Part model, mm, in its own coordinate system. A direction names the side the tool comes from. Give positions to 0.01 mm unless a question says otherwise; leave off trailing zeros. Order: outer loops, then holes, each group sorted by start corner. A loop starts at its lowest first (then second) coordinate and runs counter-clockwise, first axis right, second up. Notation, with made-up numbers: (7, 7) - (28, 7) arc R21 ccw to (28, 24) - close; hole circle Ø8 at (-27.75, 85). An arc over 180 degrees is marked (long way). One line per item, written item: value.
```python
from build123d import *

# Parameters (mm, degrees)
SKETCH1_R                = 24.5
SKETCH1_R_2              = 22
BOSS_EXTRUDE1_DEPTH      = 1
BOSS_EXTRUDE2_DEPTH      = 1
SKETCH3_R                = 7
CUT_EXTRUDE1_DEPTH       = 0.9
FILLET1_R                = 0.5
BOSS_EXTRUDE3_DEPTH      = 4
BOSS_EXTRUDE3_DEPTH_BACK = 21.5
SKETCH4_R                = 28.5
SKETCH4_R_2              = 24.5
BOSS_EXTRUDE4_DEPTH      = 8
SKETCH6_R                = 4.6
BOSS_EXTRUDE5_DEPTH      = 17.5


with BuildPart() as part:
    # Sketch1 → Boss-Extrude1 (new body)
    with BuildSketch(Plane.XY):
        Circle(SKETCH1_R)
        Circle(SKETCH1_R_2, mode=Mode.SUBTRACT)
    extrude(amount=BOSS_EXTRUDE1_DEPTH)

    # Sketch2 → Boss-Extrude2 (add)
    with BuildSketch(Plane.XY.offset(1)):
        with BuildLine():
            Line((-1.614189839, 23), (1.614189839, 23))
            ThreePointArc((1.614189839, 23), (2.986252504, 22.455143994), (3.610738586, 21.117444044))
            Line((3.610738586, 21.117444044), (4.203159318, 11.046291601))
            ThreePointArc((4.203159318, 11.046291601), (5.845115801, 8.045111712), (9.206799949, 7.410933888))
            Line((9.206799949, 7.410933888), (18.96810318, 9.959665548))
            ThreePointArc((18.96810318, 9.959665548), (20.433308247, 9.779116009), (21.375487782, 8.642576636))
            Line((21.375487782, 8.642576636), (22.373111967, 5.572205105))
            ThreePointArc((22.373111967, 5.572205105), (22.278913793, 4.098926202), (21.199662351, 3.091632627))
            Line((21.199662351, 3.091632627), (11.804495268, -0.583950228))
            ThreePointArc((11.804495268, -0.583950228), (9.457596034, -3.072959231), (9.893274614, -6.46608257))
            Line((9.893274614, -6.46608257), (15.333671053, -14.962032219))
            ThreePointArc((15.333671053, -14.962032219), (15.614731503, -16.411317921), (14.824967815, -17.658593889))
            Line((14.824967815, -17.658593889), (12.213153791, -19.556187853))
            ThreePointArc((12.213153791, -19.556187853), (10.782873453, -19.921868284), (9.491373297, -19.20671))
            Line((9.491373297, -19.20671), (3.092419978, -11.40719269))
            ThreePointArc((3.092419978, -11.40719269), (0, -9.944304962), (-3.092419978, -11.40719269))
            Line((-3.092419978, -11.40719269), (-9.491373297, -19.20671))
            ThreePointArc((-9.491373297, -19.20671), (-10.782873453, -19.921868284), (-12.213153791, -19.556187853))
            Line((-12.213153791, -19.556187853), (-14.824967815, -17.658593889))
            ThreePointArc((-14.824967815, -17.658593889), (-15.614731503, -16.411317921), (-15.333671053, -14.962032219))
            Line((-15.333671053, -14.962032219), (-9.893274614, -6.46608257))
            ThreePointArc((-9.893274614, -6.46608257), (-9.457596034, -3.072959231), (-11.804495268, -0.583950228))
            Line((-11.804495268, -0.583950228), (-21.199662351, 3.091632627))
            ThreePointArc((-21.199662351, 3.091632627), (-22.278913793, 4.098926202), (-22.373111967, 5.572205105))
            Line((-22.373111967, 5.572205105), (-21.375487782, 8.642576636))
            ThreePointArc((-21.375487782, 8.642576636), (-20.433308247, 9.779116009), (-18.96810318, 9.959665548))
            Line((-18.96810318, 9.959665548), (-9.206799949, 7.410933888))
            ThreePointArc((-9.206799949, 7.410933888), (-5.845115801, 8.045111712), (-4.203159318, 11.046291601))
            Line((-4.203159318, 11.046291601), (-3.610738586, 21.117444044))
            ThreePointArc((-3.610738586, 21.117444044), (-2.986252504, 22.455143994), (-1.614189839, 23))
        make_face()
    extrude(amount=BOSS_EXTRUDE2_DEPTH)

    # Sketch3 → Cut-Extrude1 (cut)
    with BuildSketch(Plane.XY.offset(2)):
        Circle(SKETCH3_R)
    extrude(amount=-CUT_EXTRUDE1_DEPTH, mode=Mode.SUBTRACT)

    # Fillet1
    fillet1_edges = [part.edges().sort_by_distance(p)[0] for p in [
        (-7, 0, 1.1),
    ]]
    fillet(fillet1_edges, radius=FILLET1_R)

    # Sketch4 → Boss-Extrude3 (add, two sides: drawn at the far end of the back side and taken through both)
    with BuildSketch(Plane.XY.offset(-BOSS_EXTRUDE3_DEPTH_BACK)):
        Circle(SKETCH4_R)
        Circle(SKETCH4_R_2, mode=Mode.SUBTRACT)
    extrude(amount=BOSS_EXTRUDE3_DEPTH + BOSS_EXTRUDE3_DEPTH_BACK)

    # Sketch5 → Boss-Extrude4 (add)
    with BuildSketch(Plane(origin=(0, 0, 1), x_dir=(-1, 0, 0), z_dir=(0, 0, -1))):
        with BuildLine():
            Line((22.451817346, 7.975399256), (22.851723851, 6.744613588))
            Line((22.851723851, 6.744613588), (7.30628104, 1.693593032))
            ThreePointArc((7.30628104, 1.693593032), (7.132923872, -2.317627458), (4.915436519, -5.664669789))
            Line((4.915436519, -5.664669789), (14.523048547, -18.888413283))
            Line((14.523048547, -18.888413283), (13.476079724, -19.649080658))
            Line((13.476079724, -19.649080658), (3.868467697, -6.425337165))
            ThreePointArc((3.868467697, -6.425337165), (0, -7.5), (-3.868467697, -6.425337165))
            Line((-3.868467697, -6.425337165), (-13.476079724, -19.649080658))
            Line((-13.476079724, -19.649080658), (-14.523048547, -18.888413283))
            Line((-14.523048547, -18.888413283), (-4.915436519, -5.664669789))
            ThreePointArc((-4.915436519, -5.664669789), (-7.132923872, -2.317627458), (-7.30628104, 1.693593032))
            Line((-7.30628104, 1.693593032), (-22.851723851, 6.744613588))
            Line((-22.851723851, 6.744613588), (-22.451817346, 7.975399256))
            Line((-22.451817346, 7.975399256), (-6.906374535, 2.9243787))
            ThreePointArc((-6.906374535, 2.9243787), (-4.408389392, 6.067627458), (-0.647062318, 7.472035222))
            Line((-0.647062318, 7.472035222), (-0.647062318, 23.817481096))
            Line((-0.647062318, 23.817481096), (0.647062318, 23.817481096))
            Line((0.647062318, 23.817481096), (0.647062318, 7.472035222))
            ThreePointArc((0.647062318, 7.472035222), (4.408389392, 6.067627458), (6.906374535, 2.9243787))
            Line((6.906374535, 2.9243787), (22.451817346, 7.975399256))
        make_face()
    extrude(amount=BOSS_EXTRUDE4_DEPTH)

    # Sketch6 → Boss-Extrude5 (add)
    with BuildSketch(Plane(origin=(0, 0, -7), x_dir=(-1, 0, 0), z_dir=(0, 0, -1))):
        Circle(SKETCH6_R)
        with BuildLine():
            Line((-2.436698586, -1.75), (2.436698586, -1.75))
            ThreePointArc((2.436698586, -1.75), (3, 0), (2.436698586, 1.75))
            Line((2.436698586, 1.75), (-2.436698586, 1.75))
            ThreePointArc((-2.436698586, 1.75), (-3, 0), (-2.436698586, -1.75))
        make_face(mode=Mode.SUBTRACT)
    extrude(amount=BOSS_EXTRUDE5_DEPTH)


solid = part.part
```
1) Wall check: line 1 along Y through (x, z) = (0, 1.7); line 2 along Y through (x, z) = (0, -10); line 3 along Y through (x, z) = (0, -6). Give the ranges that are in metal, low to high. Write a range as [from, to].
Answer:
line 1: y = [-28.5, -24.5], [-9.94, -7], [7, 23], [24.5, 28.5]
line 2: y = [-28.5, -24.5], [-4.6, -1.75], [1.75, 4.6], [24.5, 28.5]
line 3: y = [-28.5, -24.5], [-7.5, 23.82], [24.5, 28.5]
2) Two-plate mould, pull along Y, no slides. Class faces 1 (the face through (13, 21, -21.5)), 2 (the face through (0, 0, -7)): pulls with the +Y half, pulls with the -Y half, needs draft (parallel to the pull), parting line crosses it, or undercut.
Answer:
face 1: needs draft
face 2: undercut
3) Slice it at D-D on y = 17. Write the cut outline in (x, z).
Answer:
outline: (-22.87, -21.5) - (-17.64, -21.5) - (-17.64, 0) - (-13.96, 0) - (-13.96, 1) - (-17.64, 1) - (-17.64, 4) - (-22.87, 4) - close; (-3.85, 1) - (-0.65, 1) - (-0.65, -7) - (0.65, -7) - (0.65, 1) - (3.85, 1) - (3.85, 2) - (-3.85, 2) - close; (13.96, 0) - (17.64, 0) - (17.64, -21.5) - (22.87, -21.5) - (22.87, 4) - (17.64, 4) - (17.64, 1) - (13.96, 1) - close
4) Slice it at A-A on z = -2.5. Write the cut outline in (x, y).
Answer:
outline: circle Ø57 at (0, 0); (-22.85, 6.74) - (-7.31, 1.69) arc R7.5 ccw to (-4.92, -5.66) - (-14.52, -18.89) - (-13.48, -19.65) - (-3.87, -6.43) arc R7.5 ccw to (3.87, -6.43) - (13.48, -19.65) - (14.52, -18.89) - (4.92, -5.66) arc R7.5 ccw to (7.31, 1.69) - (22.85, 6.74) - (22.45, 7.98) - (6.91, 2.92) arc R7.5 ccw to (0.65, 7.47) - (0.65, 23.82) - (-0.65, 23.82) - (-0.65, 7.47) arc R7.5 ccw to (-6.91, 2.92) - (-22.45, 7.98) - close; hole circle Ø49 at (0, 0)
5) Slice it at B-B on z = -18.5. Write the cut outline in (x, y), then the cut area to 3 significant figures.
Answer:
outline: circle Ø57 at (0, 0); circle Ø9.2 at (0, 0); hole circle Ø49 at (0, 0); hole (-2.44, -1.75) - (2.44, -1.75) arc R3 ccw to (2.44, 1.75) - (-2.44, 1.75) arc R3 ccw to start
area: 713 mm2
6) Drop flat-ended pins along their axis: P1, Ø17, axis at x = 5.5, y = -13.5, coming from the -Z side; P2, Ø8.5, axis at x = 0, y = 0, coming from the +Z side; P3, Ø5, axis at x = -12, y = -6.5, coming from the +Z side. Give the stop position or say it passes through.
Answer:
P1: stops at z = -7
P2: stops at z = 1.1
P3: stops at z = 2
7) Slice it at C-C on x = -17.5. Write the cut outline in (y, z), then the cut area to 3 significant figures.
Answer:
outline: (-22.49, -21.5) - (-17.15, -21.5) - (-17.15, 0) - (-13.33, 0) - (-13.33, 1) - (-17.15, 1) - (-17.15, 4) - (-22.49, 4) - close; (1.64, 1) - (5.01, 1) - (5.01, -7) - (6.37, -7) - (6.37, 1) - (9.58, 1) - (9.58, 2) - (1.64, 2) - close; (13.33, 0) - (17.15, 0) - (17.15, -21.5) - (22.49, -21.5) - (22.49, 4) - (17.15, 4) - (17.15, 1) - (13.33, 1) - close
area: 299 mm2
8) Which spindle directions (+Z, -Z, +X, -X, +Y, -Y) get a long thin tool onto all of the face, cutting with end or side? Do faces 3 (the face through (0, 23.817, -3)), 4 (the face through (-16.44, 1.23, 1.49)), 5 (the face through (13, 21, 4)), 6 (the face through (0, 0, 1.1)). Say none if no direction does.
Answer:
face 3: -Z
face 4: +Z, -Z
face 5: +Z, +X, -X, +Y, -Y
face 6: +Z
